from build123d import *

# Parameters (mm, degrees)
SKETCH_R        = 52
SKETCH_R_2      = 4
PAD_DEPTH       = 3
SKETCH001_R     = 45
SKETCH001_R_2   = 40.5
PAD001_DEPTH    = 12
SKETCH002_R     = 2.5
POCKET_DEPTH    = 3.001
SKETCH003_R     = 17
SKETCH003_R_2   = 12.5
PAD002_DEPTH    = 6
SKETCH004_R     = 6
SKETCH004_R_2   = 4
PAD003_DEPTH    = 5
CHAMFER_SIZE    = 1.5
CHAMFER001_SIZE = 1
CHAMFER002_SIZE = 0.6
SKETCH005_R     = 1.6
POCKET001_DEPTH = 3.001


with BuildPart() as part:
    # Sketch → Pad (new body)
    with BuildSketch(Plane.XY):
        Circle(SKETCH_R)
        Circle(SKETCH_R_2, mode=Mode.SUBTRACT)
    extrude(amount=PAD_DEPTH)

    # Sketch001 (on Face4 of Pad) → Pad001 (join)
    with BuildSketch(Plane.XY.offset(3)):
        Circle(SKETCH001_R)
        Circle(SKETCH001_R_2, mode=Mode.SUBTRACT)
    extrude(amount=PAD001_DEPTH)

    # Sketch002 (on Face6 of Pad001) → Pocket (cut, through all)
    with BuildSketch(Plane.XY.offset(3)):
        with Locations((-30.5, 5)):
            Circle(SKETCH002_R)
        with Locations((-30.5, -15)):
            Circle(SKETCH002_R)
        with Locations((-10.5, -25)):
            Circle(SKETCH002_R)
        with Locations((9.5, 25)):
            Circle(SKETCH002_R)
        with Locations((29.5, 15)):
            Circle(SKETCH002_R)
        with Locations((29.5, -5)):
            Circle(SKETCH002_R)
    extrude(amount=-POCKET_DEPTH, mode=Mode.SUBTRACT)

    # Sketch003 (on Face12 of Pocket) → Pad002 (join)
    with BuildSketch(Plane.XY.offset(3)):
        Circle(SKETCH003_R)
        Circle(SKETCH003_R_2, mode=Mode.SUBTRACT)
    extrude(amount=PAD002_DEPTH)

    # Sketch004 (on Face13 of Pad002) → Pad003 (join)
    with BuildSketch(Plane.XY.offset(3)):
        Circle(SKETCH004_R)
        Circle(SKETCH004_R_2, mode=Mode.SUBTRACT)
    extrude(amount=PAD003_DEPTH)

    # Chamfer
    chamfer_edges = [part.edges().sort_by_distance(p)[0] for p in [
        (-45, 0, 15),
    ]]
    chamfer(chamfer_edges, length=CHAMFER_SIZE)

    # Chamfer001
    chamfer001_edges = [part.edges().sort_by_distance(p)[0] for p in [
        (-12.5, 0, 9),
    ]]
    chamfer(chamfer001_edges, length=CHAMFER001_SIZE)

    # Chamfer002
    chamfer002_edges = [part.edges().sort_by_distance(p)[0] for p in [
        (-6, 0, 8),
    ]]
    chamfer(chamfer002_edges, length=CHAMFER002_SIZE)

    # Sketch005 (on Face19 of Chamfer002) → Pocket001 (cut, through all)
    with BuildSketch(Plane.XY.offset(3)):
        with Locations((-24.792704, 27.46492)):
            Circle(SKETCH005_R)
        with Locations((36.18167, 7.738652)):
            Circle(SKETCH005_R)
        with Locations((-11.388966, -35.203572)):
            Circle(SKETCH005_R)
    extrude(amount=-POCKET001_DEPTH, mode=Mode.SUBTRACT)


solid = part.part
Work out the finished part from the listing and answer in its coordinate system (mm). A direction names the side the tool comes from. Round coordinates to 2 decimals unless told otherwise and drop trailing zeros. Loops run counter-clockwise (first coordinate to the right, second up) from the corner with the lowest first, then second, coordinate; pieces in that order, holes last. Notation, with made-up numbers: (67.5, -37.5) - (111.5, -37.5) arc R21 cw to (111.5, -21.5) - close; hole circle Ø11 at (-28, -24.75). An arc over 180 degrees is marked (long way). Use one line per item in the form item = value. Start each with the question number.
(1) Find section D-D on x = -30.5. Give the number of separate pieces and of enclosed holes in the cut face, and give its area (3 significant figures).
(2) Which of the six approach directions +Z, -Z, +X, -X, +Y, -Y give full straight-line access (tool end or side, diameter ignored) to faces 4 (the face through (-4, -2, 8)), 5 (the face through (37.66, 7.13, 1.52))?
(3) Determine the mould class of faces 1 (the face through (5.4, 3, 3)), 2 (the face through (-41.265, -31.641, 1.479)), 3 (the face through (11, 1, 0)) for opening direction Y: +Y half, -Y half, draft (parallel to the pull), parting line (faces both ways), or undercut.
(4) Flat-ended cylindrical pins translate along their axes: P1, Ø8, axis at y = -41, z = 6.5, coming from the +X side; P2, Ø2, axis at x = -40, z = 9.5, coming from the +Y side; P3, Ø2, axis at y = 9, z = 12.5, coming from the -X side; P4, Ø1.9, axis at x = 36.18, y = 7.74, coming from the -Z side. Find the tip coordinate at first contact, or state that the pin passes through.
(5) Consider line 1 (Y direction, x = 0, z = 11); line 2 (X direction, y = 11.5, z = 6); line 3 (X direction, y = 6, z = 8.25). Determine where each line is inside the solid, lowest interval first.
(6) Find section C-C on z = 10.5. Determine the outline of the cut face in (x, y).
Answer list:
q1.separate_pieces = 3
q1.enclosed_holes = 0
q1.area = 374 mm^2
q2.face_4 = +Z
q2.face_5 = +Z, -Z
q3.face_1 = undercut
q3.face_2 = parting line
q3.face_3 = draft
q4.P1 = 34.32
q4.P2 = 22.45
q4.P3 = -44.28
q4.P4 = through
q5.line_1 = -45 to -40.5, 40.5 to 45
q5.line_2 = -43.51 to -38.83, -12.52 to -4.9, 4.9 to 12.52, 38.83 to 43.51
q5.line_3 = -44.6 to -40.05, -15.91 to -11.25, 11.25 to 15.91, 40.05 to 44.6
q6.outline = circle Ø90 at (0, 0); hole circle Ø81 at (0, 0)
